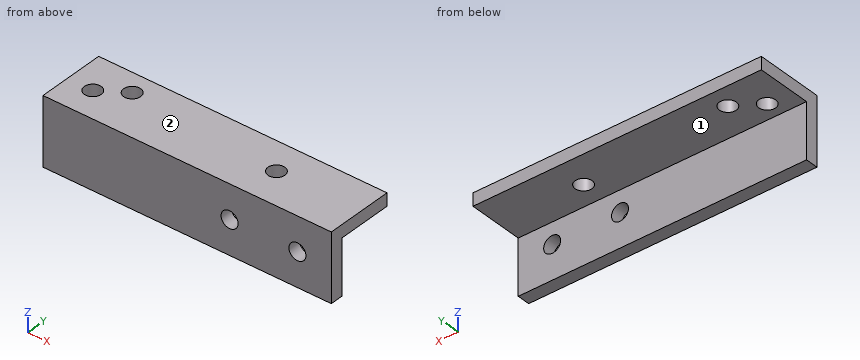
from build123d import *

# Parameters (mm, degrees)
BOSS_EXTRUDE1_DEPTH = 107.95
CUT_EXTRUDE1_REACH  = 114.802
SKETCH3_R           = 3.175
CUT_EXTRUDE2_REACH  = 115.77
SKETCH4_R           = 3.175
CUT_EXTRUDE4_REACH  = 115.77
SKETCH5_R           = 3.175


with BuildPart() as part:
    # Sketch1 → Boss-Extrude1 (new body)
    with BuildSketch(Plane(origin=(0, 0, 0), x_dir=(0, 0, -1), z_dir=(1, 0, 0))):
        Polygon((0, 0), (0, -25.4), (25.4, -25.4), (25.4, -20.6375), (4.7625, -20.6375), (4.7625, 0), align=None)
    extrude(amount=BOSS_EXTRUDE1_DEPTH)

    # Sketch3 → Cut-Extrude1 (cut, up to next)
    with BuildSketch(Plane(origin=(0, 0, -4.7625), x_dir=(-1, 0, 0), z_dir=(0, 0, -1)), mode=Mode.PRIVATE) as cut_extrude1_sk1:
        with Locations(Location((-9.525, -14.2875, 0), (0, 0, 90))):
            Circle(SKETCH3_R)
    cut_extrude1_tool1 = extrude(cut_extrude1_sk1.sketch, amount=-CUT_EXTRUDE1_REACH, mode=Mode.PRIVATE) & part.part
    # Sketch3 → Cut-Extrude1 (cut, up to next)
    with BuildSketch(Plane(origin=(0, 0, -4.7625), x_dir=(-1, 0, 0), z_dir=(0, 0, -1)), mode=Mode.PRIVATE) as cut_extrude1_sk2:
        with Locations(Location((-19.05, -7.9375, 0), (0, 0, 90))):
            Circle(SKETCH3_R)
    cut_extrude1_tool2 = extrude(cut_extrude1_sk2.sketch, amount=-CUT_EXTRUDE1_REACH, mode=Mode.PRIVATE) & part.part
    add(cut_extrude1_tool1.solids().sort_by_distance((9.525, -14.2875, -4.7625))[0], mode=Mode.SUBTRACT)
    add(cut_extrude1_tool2.solids().sort_by_distance((19.05, -7.9375, -4.7625))[0], mode=Mode.SUBTRACT)

    # Sketch4 → Cut-Extrude2 (cut, up to next)
    with BuildSketch(Plane.XY, mode=Mode.PRIVATE) as cut_extrude2_sk1:
        with Locations((76.332177029, -11.929615818)):
            Circle(SKETCH4_R)
    cut_extrude2_tool1 = extrude(cut_extrude2_sk1.sketch, amount=-CUT_EXTRUDE2_REACH, mode=Mode.PRIVATE) & part.part
    add(cut_extrude2_tool1.solids().sort_by_distance((76.332177, -11.929616, 0))[0], mode=Mode.SUBTRACT)

    # Sketch5 → Cut-Extrude4 (cut, up to next)
    with BuildSketch(Plane.XZ.offset(25.4), mode=Mode.PRIVATE) as cut_extrude4_sk1:
        with Locations(Location((69.85, -12.7, 0), (0, 0, 270))):
            Circle(SKETCH5_R)
    cut_extrude4_tool1 = extrude(cut_extrude4_sk1.sketch, amount=-CUT_EXTRUDE4_REACH, mode=Mode.PRIVATE) & part.part
    # Sketch5 → Cut-Extrude4 (cut, up to next)
    with BuildSketch(Plane.XZ.offset(25.4), mode=Mode.PRIVATE) as cut_extrude4_sk2:
        with Locations(Location((95.25, -12.7, 0), (0, 0, 270))):
            Circle(SKETCH5_R)
    cut_extrude4_tool2 = extrude(cut_extrude4_sk2.sketch, amount=-CUT_EXTRUDE4_REACH, mode=Mode.PRIVATE) & part.part
    add(cut_extrude4_tool1.solids().sort_by_distance((69.85, -25.4, -12.7))[0], mode=Mode.SUBTRACT)
    add(cut_extrude4_tool2.solids().sort_by_distance((95.25, -25.4, -12.7))[0], mode=Mode.SUBTRACT)


solid = part.part
The listing builds one solid part. Answer for the finished solid, in the listing's coordinates (mm). Face numbers are marked on the shaded views. A direction names the side the tool comes from. Give positions to 0.01 mm unless a question says otherwise; leave off trailing zeros. Write each loop counter-clockwise with the first axis right and the second up, starting at its lowest first coordinate (ties: lowest second). Pieces come first, ordered by that corner, then holes. Notation, with made-up numbers: (3.5, 36) -> (38.5, 36) arc R9 ccw to (38.5, 53) -> close; hole circle Ø1 at (71.25, 47.5). An arc over 180 degrees is marked (long way). One line per question, with ' | ' between items. Start each with the question number.
1. Section A-A (z = -12.7) is taken. State how many separate pieces and enclosed holes the cut face has, plus the area to 3 significant figures.
2. Section D-D (x = 42) is taken. Determine the outline of the cut face in (y, z).
3. Section C-C (y = -9.75) is taken. Determine the outline of the cut face in (x, z).
4. For the marked faces 1 and 2, determine the directions among +Z, -Z, +X, -X, +Y, -Y from which every point of the face is accessible in a straight line to the end or side of a thin tool.
5. Find the intervals of material crossed by probe 1 along X at (y, z) = (-23.9, -12.7) (3 decimals); probe 2 along X at (y, z) = (-14, -3.75); probe 3 along Y at (x, z) = (91.5, -7), in increasing order.
6. Section B-B (x = 19.05) is taken. Determine the outline of the cut face in (y, z).
7. Given pin 1 Ø1.5 at (x, z) = (49.5, -13) entering from +Y; pin 2 Ø6 at (x, y) = (75, -9) entering from -Z, each flat-ended and moving along its own axis, determine where each tip first touches the part or whether it passes through.
Response values:
1) separate pieces: 3 | enclosed holes: 0 | area: 454 mm2
2) outline: (-25.4, -25.4) -> (-20.64, -25.4) -> (-20.64, -4.76) -> (0, -4.76) -> (0, 0) -> (-25.4, 0) -> close
3) outline: (0, -4.76) -> (16.44, -4.76) -> (16.44, 0) -> (0, 0) -> close; (21.66, -4.76) -> (74.02, -4.76) -> (74.02, 0) -> (21.66, 0) -> close; (78.64, -4.76) -> (107.95, -4.76) -> (107.95, 0) -> (78.64, 0) -> close
4) face 1: -Z, +X, -X, +Y | face 2: +Z, +X, -X, +Y, -Y
5) probe 1: 0 to 66.675, 73.025 to 92.075, 98.425 to 107.95 | probe 2: 0 to 6.36, 12.69 to 73.93, 78.74 to 107.95 | probe 3: -25.4 to -20.64
6) outline: (-25.4, -25.4) -> (-20.64, -25.4) -> (-20.64, -4.76) -> (-11.11, -4.76) -> (-11.11, 0) -> (-25.4, 0) -> close; (-4.76, -4.76) -> (0, -4.76) -> (0, 0) -> (-4.76, 0) -> close
7) pin 1: y = -20.64 | pin 2: z = -4.76
